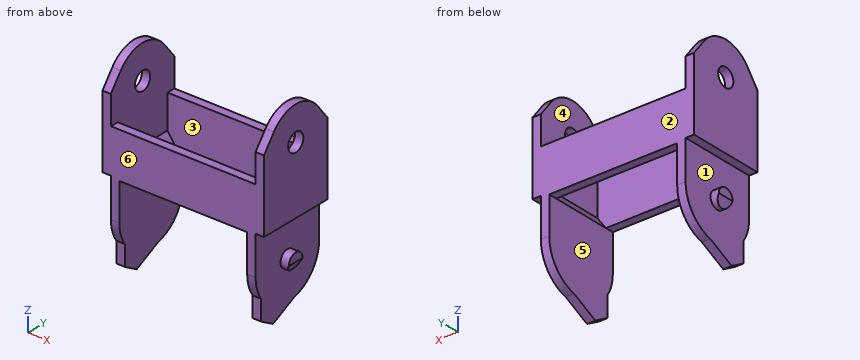
```python
from build123d import *

# Parameters (mm, degrees)
BOSS_EXTRUDE1_DEPTH = 24
SKETCH2_W           = 23
SKETCH2_H           = 23
CUT_EXTRUDE1_DEPTH  = 2.5
SKETCH4_W           = 43
SKETCH4_H           = 17
CUT_EXTRUDE2_DEPTH  = 44.462627624
SKETCH5_W           = 38
SKETCH5_H           = 22.5
CUT_EXTRUDE3_DEPTH  = 44.462627624
CUT_EXTRUDE4_DEPTH  = 9
SKETCH7_R           = 2.75
CUT_EXTRUDE5_DEPTH  = 57.747246629
SKETCH8_R           = 2.5
BOSS_EXTRUDE2_DEPTH = 2.5
CUT_EXTRUDE6_DEPTH  = 44.462627624
BOSS_EXTRUDE4_DEPTH = 2.5


with BuildPart() as part:
    # Sketch1 → Boss-Extrude1 (new, symmetric)
    with BuildSketch(Plane(origin=(0, 0, 0), x_dir=(0, 0, -1), z_dir=(1, 0, 0))):
        with BuildLine():
            Line((16.5, -11.5), (-16.5, -11.5))
            Line((-16.5, -11.5), (-21.137338715, -7.895129733))
            ThreePointArc((-21.137338715, -7.895129733), (-25, 0), (-21.137338715, 7.895129733))
            Line((-21.137338715, 7.895129733), (-16.5, 11.5))
            Line((-16.5, 11.5), (16.5, 11.5))
            ThreePointArc((16.5, 11.5), (28, 0), (16.5, -11.5))
        make_face()
    extrude(amount=BOSS_EXTRUDE1_DEPTH, both=True)

    # Sketch2 → Cut-Extrude1 (cut)
    with BuildSketch(Plane(origin=(24, 0, 0), x_dir=(0, 0, -1), z_dir=(1, 0, 0))):
        with Locations((16.5, 0)):
            Rectangle(SKETCH2_W, SKETCH2_H)
    cut_extrude1 = extrude(amount=-CUT_EXTRUDE1_DEPTH, mode=Mode.SUBTRACT)

    # Mirror1: Cut-Extrude1 across plane
    add(cut_extrude1.mirror(Plane(origin=(0, 0, 0), x_dir=(0, 0, 1), z_dir=(1, 0, 0))), mode=Mode.SUBTRACT)

    # Sketch4 → Cut-Extrude2 (cut, through all)
    with BuildSketch(Plane(origin=(0, 11.5, 0), x_dir=(1, 0, 0), z_dir=(0, 1, 0))):
        with Locations((0, -16.5)):
            Rectangle(SKETCH4_W, SKETCH4_H)
    extrude(amount=-CUT_EXTRUDE2_DEPTH, mode=Mode.SUBTRACT)

    # Sketch5 → Cut-Extrude3 (cut, through all)
    with BuildSketch(Plane(origin=(0, 11.5, 0), x_dir=(1, 0, 0), z_dir=(0, 1, 0))):
        with Locations((0, 16.75)):
            Rectangle(SKETCH5_W, SKETCH5_H)
    extrude(amount=-CUT_EXTRUDE3_DEPTH, mode=Mode.SUBTRACT)

    # Sketch6 → Cut-Extrude4 (cut, symmetric)
    with BuildSketch(Plane(origin=(0, 0, 0), x_dir=(1, 0, 0), z_dir=(0, 1, 0))):
        Polygon((-19, 5.5), (-21.5, 2), (-21.5, -8), (21.5, -8), (21.5, 2), (19, 5.5), align=None)
    extrude(amount=CUT_EXTRUDE4_DEPTH, both=True, mode=Mode.SUBTRACT)

    # Sketch7 → Cut-Extrude5 (cut, through all)
    with BuildSketch(Plane(origin=(24, 0, 0), x_dir=(0, 0, -1), z_dir=(1, 0, 0))):
        with Locations((-15, 0)):
            Circle(SKETCH7_R)
    extrude(amount=-CUT_EXTRUDE5_DEPTH, mode=Mode.SUBTRACT)

    # Sketch8 → Boss-Extrude2 (add, through all)
    with BuildSketch(Plane(origin=(21.5, 0, 0), x_dir=(0, 0, -1), z_dir=(1, 0, 0))):
        with Locations((16.5, 0)):
            Circle(SKETCH8_R)
    boss_extrude2 = extrude(amount=BOSS_EXTRUDE2_DEPTH)

    # Sketch9 → Cut-Extrude6 (cut, through all)
    with BuildSketch(Plane(origin=(0, 11.5, 0), x_dir=(1, 0, 0), z_dir=(0, 1, 0))):
        Polygon((22.75, 19), (24, 16.5), (24, 19), align=None)
    cut_extrude6 = extrude(amount=-CUT_EXTRUDE6_DEPTH, mode=Mode.SUBTRACT)

    # Sketch10 → Boss-Extrude4 (add)
    with BuildSketch(Plane(origin=(21.5, 0, 0), x_dir=(0, 0, -1), z_dir=(1, 0, 0))):
        with BuildLine():
            Line((27.72497216, 2.5), (31.5, -5.181049598))
            Line((31.5, -5.181049598), (28.980740698, -9.5))
            Line((28.980740698, -9.5), (22.980740698, -9.5))
            ThreePointArc((22.980740698, -9.5), (27.194534443, -4.228112231), (27.72497216, 2.5))
        make_face()
    boss_extrude4 = extrude(amount=-BOSS_EXTRUDE4_DEPTH)

    # Mirror2: Boss-Extrude2, Cut-Extrude6, Boss-Extrude4 across plane
    add(boss_extrude2.mirror(Plane(origin=(0, 0, 0), x_dir=(0, 0, 1), z_dir=(1, 0, 0))))
    add(cut_extrude6.mirror(Plane(origin=(0, 0, 0), x_dir=(0, 0, 1), z_dir=(1, 0, 0))), mode=Mode.SUBTRACT)
    add(boss_extrude4.mirror(Plane(origin=(0, 0, 0), x_dir=(0, 0, 1), z_dir=(1, 0, 0))))


solid = part.part
```
CAD build for the part. Positions are in the model's coordinates, mm. Face numbers are marked on the shaded views. A direction names the side the tool comes from. Round coordinates to 2 decimals unless told otherwise and drop trailing zeros. Order: outer loops, then holes, each group sorted by start corner. A loop starts at its lowest first (then second) coordinate and runs counter-clockwise, first axis right, second up.
Q1. Slice it at A-A (z = 15). Write the cut outline in (x, y), and give its area (3 significant figures).
Q2. Slice it at C-C (z = -25.5). Write the cut outline in (x, y), and give its area (3 significant figures).
Q3. Which spindle directions (+Z, -Z, +X, -X, +Y, -Y) get a long thin tool onto all of the face, cutting with end or side? Do the marked faces 4, 5 and 6. Say none if no direction does.
Q4. Drop flat-ended pins along their axis: pin 1 (4 mm diameter, centred on y = -8.5, z = -23, fed in from -X); pin 2 (3 mm diameter, centred on x = 20.5, z = -25.5, fed in from -Y); pin 3 (5 mm diameter, centred on x = -11.5, y = -9, fed in from +Z); pin 4 (1 mm diameter, centred on x = 18, z = -14, fed in from -Y). Give the stop position or say it passes through.
Q5. Two-plate mould, pull along Y, no slides. Class the marked faces 1, 2 and 3: pulls with the +Y half, pulls with the -Y half, needs draft (parallel to the pull), parting line crosses it, or undercut.
Q6. Wall check: L1, parallel to X at y = 9.75, z = -22.5; L2, parallel to X at y = 2.75, z = 10; L3, parallel to Y at x = 3, z = 4.5. Give the ranges that are in metal, low to high.
Q7. Slice it at B-B (x = 0). Write the cut outline in (y, z).
Q8. Slice it at D-D (y = -4.25). Write the cut outline in (x, z).
Results below:
1. outline: (-24, -11.5) - (-21.5, -11.5) - (-21.5, -2.75) - (-24, -2.75) - close; (-24, 2.75) - (-21.5, 2.75) - (-21.5, 11.5) - (-24, 11.5) - close; (21.5, -11.5) - (24, -11.5) - (24, -2.75) - (21.5, -2.75) - close; (21.5, 2.75) - (24, 2.75) - (24, 11.5) - (21.5, 11.5) - close
1. area: 87.5 mm2
2. outline: (-21.5, -9.5) - (-19, -9.5) - (-19, 7.16) - (-21.5, 7.16) - close; (19, -9.5) - (21.5, -9.5) - (21.5, 7.16) - (19, 7.16) - close
2. area: 83.3 mm2
3. face 4: +Z
3. face 5: -Z, +Y, -Y
3. face 6: +Z, -Z, +X, -X, -Y
4. pin 1: stops at x = -21.5
4. pin 2: stops at y = -9.5
4. pin 3: stops at z = 8
4. pin 4: passes through
5. face 1: needs draft
5. face 2: pulls with the +Y half
5. face 3: undercut
6. L1: x = -21.5 to -19, 19 to 21.5
6. L2: x = -24 to -21.5, 21.5 to 24
6. L3: y = -11.5 to -9, 9 to 11.5
7. outline: (-11.5, -5.5) - (-9, -5.5) - (-9, 8) - (-11.5, 8) - close; (9, -5.5) - (11.5, -5.5) - (11.5, 8) - (9, 8) - close
8. outline: (-24, -5) - (-21.5, -5) - (-21.5, -31.04) - (-19, -31.04) - (-19, -5.5) - (-21.5, -2) - (-21.5, 24.05) - (-24, 24.05) - close; (19, -31.04) - (21.5, -31.04) - (21.5, -5) - (24, -5) - (24, 24.05) - (21.5, 24.05) - (21.5, -2) - (19, -5.5) - close
